Geometry check sheet. Reference: the model listing, model coordinates, mm. A direction names the side the tool comes from. Give positions to 0.01 mm unless a question says otherwise; leave off trailing zeros. Write each loop counter-clockwise with the first axis right and the second up, starting at its lowest first coordinate (ties: lowest second). Pieces come first, ordered by that corner, then holes.
(1) Depth check by flat-ended pin: P1, Ø5.5, axis at y = 104.5, z = 16.5, coming from the -X side; P2, Ø1.6, axis at y = 83, z = 16, coming from the +X side; P3, Ø16, axis at x = 138.7, y = 15, coming from the +Z side; P4, Ø22, axis at x = 141.5, z = 8.5, coming from the -Y side. Enter the tip coordinate at first touch or a pass-through.
(2) Cross-section at A-A (y = 185.5). Record the boundary of the cut face in (x, z), and give its area (3 significant figures).
(3) Cross-section at D-D (y = 15). Record the boundary of the cut face in (x, z), and give its area (3 significant figures).
(4) Thickness scan on line 1 along Y through (x, z) = (-52.5, 100); line 2 along Y through (x, z) = (-17.5, 232.5); line 3 along Z through (x, y) = (14, 210). Record the ranges inside material, lowest first.
(5) Cross-section at C-C (x = 0). Record the boundary of the cut face in (y, z), and give its area (3 significant figures).
(6) Cross-section at B-B (x = -65). Record the boundary of the cut face in (y, z), and give its area (3 significant figures).
(7) Mould release check, pull along Y, two halves, no side actions. Record for faces 1 (the flat face through (1, 24, 366)), 2 (the flat face through (1, 0, 201)), 3 (the cylindrical face through (129.467, 11.17, 9.86)): +Y half, -Y half, draft (parallel to the pull), parting line (faces both ways), or undercut.
(8) Tool access check on faces 4 (the flat face through (-20, 12, 210)), 5 (the flat face through (-137, 210, 10)), 6 (the flat face through (138, 210, 10)), 7 (the flat face through (-1, 48, 371)), 8 (the flat face through (-80, 24, 371)). Record the directions out of +Z, -Z, +X, -X, +Y, -Y that give a thin tool (end or side, any length) a straight path to the whole face; none if there is none.
```python
from build123d import *

# Parameters (mm, degrees)
EXTRUDE_1_DEPTH      = 20
EXTRUDE_2_REACH      = 387.225
EXTRUDE_2_END_RADIUS = 118.5
SKETCH_4_W           = 40
SKETCH_4_H           = 9
EXTRUDE_3_DEPTH      = 200
EXTRUDE_5_DEPTH      = 20
RIB_6_REACH          = 455.87
SKETCH_10_WALL_W     = 992.30498819
SKETCH_10_WALL_H     = 10
EXTRUDE_6_DEPTH      = 10
EXTRUDE_7_DEPTH      = 20
SKETCH_13_R          = 10
CUT_EXTRUDE_1_DEPTH  = 20
CUT_EXTRUDE_2_DEPTH  = 240
CUT_EXTRUDE_3_REACH  = 452.258
SKETCH_15_W          = 160
SKETCH_15_H          = 0.725633759


with BuildPart() as part:
    # 草图1 → 凸台-拉伸1 (new body)
    with BuildSketch(Plane(origin=(0, 0, 0), x_dir=(1, 0, 0), z_dir=(0, 1, 0))):
        with BuildLine():
            Line((-118.5, 0), (-108.5, 0))
            ThreePointArc((-108.5, 0), (0, -108.5), (108.5, 0))
            Line((108.5, 0), (118.5, 0))
            ThreePointArc((118.5, 0), (0, -118.5), (-118.5, 0))
        make_face()
    extrude(amount=EXTRUDE_1_DEPTH)

    # 凸台-拉伸2: up to this cylinder (the profile starts outside it)
    extrude_2_end = Plane(origin=(0, 10, 0), z_dir=(0, -1, 0)) * Cylinder(EXTRUDE_2_END_RADIUS, 1012.45, mode=Mode.PRIVATE)
    # 草图3 → 凸台-拉伸2 (add, up to the surface)
    with BuildSketch(Plane.XY.offset(366), mode=Mode.PRIVATE) as extrude_2_sk1:
        Polygon((0, 0), (20, 0), (20, 20), (-20, 20), (-20, 0), align=None)
    extrude_2_tool1 = extrude(extrude_2_sk1.sketch, amount=-EXTRUDE_2_REACH, mode=Mode.PRIVATE) - extrude_2_end
    add(extrude_2_tool1.solids().sort_by_distance((0, 10, 366))[0])

    # 草图4 → 凸台-拉伸3 (add)
    with BuildSketch(Plane(origin=(0, 20, 0), x_dir=(1, 0, 0), z_dir=(0, 1, 0))):
        with Locations((0, -114)):
            Rectangle(SKETCH_4_W, SKETCH_4_H)
    extrude(amount=EXTRUDE_3_DEPTH)

    # 草图5 → 凸台-拉伸5 (add)
    with BuildSketch(Plane(origin=(0, 220, 0), x_dir=(1, 0, 0), z_dir=(0, 1, 0))):
        with BuildLine():
            Line((-120.175912728, 0), (-108.5, 0))
            ThreePointArc((-108.5, 0), (0, -108.5), (108.5, 0))
            Line((108.5, 0), (120.175912728, 0))
            ThreePointArc((120.175912728, 0), (0, -120.175912728), (-120.175912728, 0))
        make_face()
    extrude(amount=EXTRUDE_5_DEPTH)

    # 草图10 wall → 筋6 (add, up to next)
    with BuildSketch(Plane(origin=(0, 51.594277654, 145.071057526), x_dir=(0, -0.765324590967, 0.643644521814), z_dir=(0, -0.643644521814, -0.765324590967)), mode=Mode.PRIVATE) as rib_6_sk1:
        Rectangle(SKETCH_10_WALL_W, SKETCH_10_WALL_H)
    rib_6_tool1 = extrude(rib_6_sk1.sketch, amount=RIB_6_REACH, mode=Mode.PRIVATE) - part.part
    add(rib_6_tool1.solids().sort_by_distance((0, 51.594277654, 145.071057526))[0])

    # 草图11 → 凸台-拉伸6 (add)
    with BuildSketch(Plane.XY.offset(366)):
        Polygon((-80, 48), (80, 48), (80, 38), (80, 20), (80, 0), (-80, 0), (-80, 20), (-80, 38), align=None)
    extrude(amount=EXTRUDE_6_DEPTH)

    # 草图12 → 凸台-拉伸7 (add)
    with BuildSketch(Plane.XY):
        Polygon((-109, 0), (-156.5, 0), (-156.5, 30), (-118.5, 30), (-118.5, 210), (-156.5, 210), (-156.5, 240), (-109, 240), align=None)
        Polygon((156.5, 0), (109, 0), (109, 240), (156.5, 240), (156.5, 210), (118.5, 210), (118.5, 30), (156.5, 30), align=None)
    extrude(amount=EXTRUDE_7_DEPTH)

    # 草图13 → 切除-拉伸1 (cut)
    with BuildSketch(Plane(origin=(0, 0, 0), x_dir=(-1, 0, 0), z_dir=(0, 0, -1))):
        with Locations((138.306064525, 225)):
            Circle(SKETCH_13_R)
        with Locations((138.306064525, 15)):
            Circle(SKETCH_13_R)
        with Locations((-138.70464108, 225)):
            Circle(SKETCH_13_R)
        with Locations((-138.70464108, 15)):
            Circle(SKETCH_13_R)
    extrude(amount=-CUT_EXTRUDE_1_DEPTH, mode=Mode.SUBTRACT)

    # 草图14 → 切除-拉伸2 (cut)
    with BuildSketch(Plane(origin=(0, 0, 0), x_dir=(1, 0, 0), z_dir=(0, 1, 0))):
        with BuildLine():
            Line((-110, 0), (110, 0))
            ThreePointArc((110, 0), (0, -110), (-110, 0))
        make_face()
    extrude(amount=CUT_EXTRUDE_2_DEPTH, mode=Mode.SUBTRACT)

    # 草图15 → 切除-拉伸3 (cut, up to next)
    with BuildSketch(Plane(origin=(0, 48, 0), x_dir=(1, 0, 0), z_dir=(0, 1, 0)), mode=Mode.PRIVATE) as cut_extrude_3_sk1:
        with Locations((0, -375.637183121)):
            Rectangle(SKETCH_15_W, SKETCH_15_H)
    cut_extrude_3_tool1 = extrude(cut_extrude_3_sk1.sketch, amount=-CUT_EXTRUDE_3_REACH, mode=Mode.PRIVATE) & part.part
    add(cut_extrude_3_tool1.solids().sort_by_distance((0, 48, 375.637183))[0], mode=Mode.SUBTRACT)


solid = part.part
```
Reply:
1. P1: stops at x = -118.5
1. P2: stops at x = 118.5
1. P3: passes through
1. P4: stops at y = 0
2. outline: (-118.5, 0) - (-110, 0) arc R110 cw to (-109, 14.8) - (-109, 20) - (-118.5, 20) - close; (-20, 109.5) - (-10.48, 109.5) arc R110 cw to (10.48, 109.5) - (20, 109.5) - (20, 118.5) - (-20, 118.5) - close; (109, 14.8) arc R110 cw to (110, 0) - (118.5, 0) - (118.5, 20) - (109, 20) - close
2. area: 713 mm2
3. outline: (-156.5, 0) - (-148.31, 0) - (-148.31, 20) - (-156.5, 20) - close; (-128.31, 0) - (-110, 0) arc R110 cw to (110, 0) - (128.7, 0) - (128.7, 20) - (116.8, 20) arc R118.5 ccw to (20, 116.8) - (20, 366) - (80, 366) - (80, 375.27) - (-80, 375.27) - (-80, 366) - (-20, 366) - (-20, 116.8) arc R118.5 ccw to (-116.8, 20) - (-128.31, 20) - close; (148.7, 0) - (156.5, 0) - (156.5, 20) - (148.7, 20) - close
3. area: 15,200 mm2
4. line 1: y = 0 to 20, 220 to 240
4. line 2: y = 0 to 20
4. line 3: z = 109.5 to 118.5
5. outline: (0, 110) - (240, 110) - (240, 120.18) - (220, 120.18) - (220, 118.5) - (83.19, 118.5) - (20, 171.64) - (20, 366) - (48, 366) - (48, 375.27) - (0, 375.27) - close
5. area: 9,150 mm2
6. outline: (0, 88.74) - (20, 88.74) - (20, 99.08) - (0, 99.08) - close; (0, 366) - (48, 366) - (48, 375.27) - (0, 375.27) - close; (220, 88.74) - (240, 88.74) - (240, 101.08) - (220, 101.08) - close
6. area: 899 mm2
7. face 1: draft
7. face 2: -Y half
7. face 3: undercut
8. face 4: -X
8. face 5: +Z, -Z, -X
8. face 6: +Z, -Z, +X
8. face 7: +Z, +X, -X, +Y
8. face 8: +Z, -X, +Y, -Y
